Could you check a few things on this model? Use its own coordinates, in mm. A direction names the side the tool comes from. Coordinates: 2 decimals unless noted, no trailing zeros. Loops run counter-clockwise (first coordinate to the right, second up) from the corner with the lowest first, then second, coordinate; pieces in that order, holes last. Notation, with made-up numbers: (81, -27.5) -> (118, -27.5) arc R13 cw to (118, -11.5) -> close; hole circle Ø6 at (27.25, 33). An arc over 180 degrees is marked (long way). One line per question, with ' | ' between items.
from build123d import *

# Parameters (mm, degrees)
F0_R     = 9.625
F1_DEPTH = 1.5875
F2_R     = 9.625
F2_R_2   = 8.0375
F3_DEPTH = 1.5875
F4_W     = 3.175
F4_H     = 12.7
F5_DEPTH = 2.38125


with BuildPart() as f1:
    # F0 (on Top) → F1 (new body)
    with BuildSketch(Plane.XY):
        Circle(F0_R)
    extrude(amount=F1_DEPTH)

    # F2 (on face) → F3 (join)
    with BuildSketch(Plane.XY.offset(1.5875)):
        Circle(F2_R)
        Circle(F2_R_2, mode=Mode.SUBTRACT)
    extrude(amount=F3_DEPTH)

    # F4 (on Top) → F5 (join)
    with BuildSketch(Plane.XY):
        with Locations((0, 15.8431801179)):
            Rectangle(F4_W, F4_H)
    extrude(amount=F5_DEPTH)


solid = f1.part
1) On a 3-axis mill with a long thin cutter (end or side, diameter ignored), from which of +Z, -Z, +X, -X, +Y, -Y can I reach the whole of each face in a straight line? I mean faces 4 (the face through (-1.588, 16, 1)), 5 (the face through (4.32, 6.78, 2.37)), 6 (the face through (1.588, 16, 1)). Say none if no direction works.
Data:
face 4: +Z, -Z, -X, +Y | face 5: +Z | face 6: +Z, -Z, +X, +Y
2) If we section it at A-A on x = 0: Please give me the cut outline in (y, z) (1 decimal), and give its area (3 significant figures).
Data:
outline: (-9.6, 0) -> (22.2, 0) -> (22.2, 2.4) -> (9.6, 2.4) -> (9.6, 3.2) -> (8, 3.2) -> (8, 1.6) -> (-8, 1.6) -> (-8, 3.2) -> (-9.6, 3.2) -> close | area: 65.5 mm²
3) I need wall thicknesses on line 1 along Y through (x, z) = (0, 2.2) (1 decimal); line 2 along Y through (x, z) = (0, 2.6) (1 decimal); line 3 along X through (y, z) = (-2.5, 2.3). Which ranges of each line are inside material? Lowest first, please. Write a range as from..to.
Data:
line 1: -9.6..-8, 8..22.2 | line 2: -9.6..-8, 8..9.6 | line 3: -9.29..-7.64, 7.64..9.29
4) If we section it at B-B on y = 0: Please give me the cut outline in (x, z) (1 decimal).
Data:
outline: (-9.6, 0) -> (9.6, 0) -> (9.6, 3.2) -> (8, 3.2) -> (8, 1.6) -> (-8, 1.6) -> (-8, 3.2) -> (-9.6, 3.2) -> close
5) I'm going to push flat-ended pins straight in: pin 1 Ø2 at (x, y) = (6, -4) entering from -Z; pin 2 Ø2.5 at (x, y) = (0.5, 15) entering from +Z; pin 3 Ø1.9 at (y, z) = (17.5, 1) entering from +X. Where does each tip first touch, or does it pass through?
Data:
pin 1: z = 0 | pin 2: z = 2.38 | pin 3: x = 1.59
6) If we section it at D-D on x = -5.25: Please give me the cut outline in (y, z) (1 decimal).
Data:
outline: (-8.1, 0) -> (8.1, 0) -> (8.1, 3.2) -> (6.1, 3.2) -> (6.1, 1.6) -> (-6.1, 1.6) -> (-6.1, 3.2) -> (-8.1, 3.2) -> close
7) We'd pull the mould along X, two halves only. Please class faces 1 (the face through (0, 0, 1.588)), 2 (the face through (-2.087, -9.396, 1.565)), 3 (the face through (0, 16, 2.381)): pulls with the +X half, pulls with the -X half, needs draft (parallel to the pull), parting line crosses it, or undercut.
Data:
face 1: undercut | face 2: parting line crosses it | face 3: needs draft
